Check sheet for the drawn part. Datum: minimum x, y, z corner. Units: mm. A direction names the side the tool comes from. Round coordinates to 2 decimals unless told otherwise and drop trailing zeros. Write each loop counter-clockwise with the first axis right and the second up, starting at its lowest first coordinate (ties: lowest second). Pieces come first, ordered by that corner, then holes. Notation, with made-up numbers: M 10.25,65 L 63.25,65 A14 cw 63.25,74 Z; hole C 52.5,32.25 d9. An arc over 180 degrees is marked long. Answer in a Markdown table with one row per item. Add a question column.
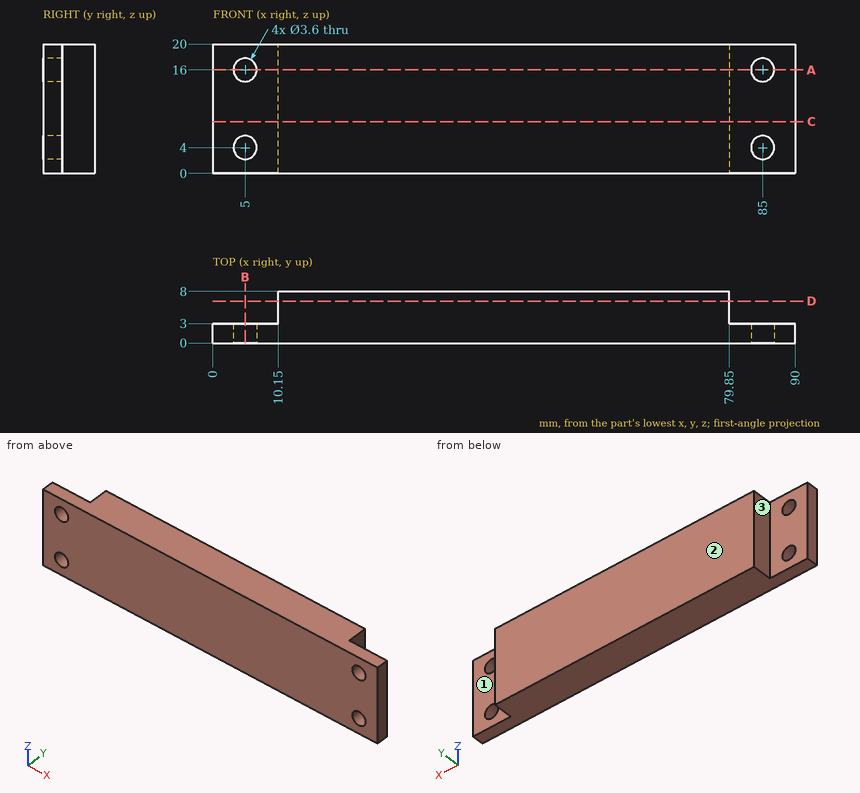
Item 1: Section check D-D, the plane y = 6.5. Record the boundary of the cut face in (x, z), and give its area (3 significant figures).
Item 2: Gauge pin test, flat ends, axial feed: pin 1 Ø2 at (x, z) = (85, 4) entering from +Y; pin 2 Ø3 at (x, z) = (85.5, 13.5) entering from +Y. Record the tip position at first contact, or that the pin passes through.
Item 3: Section check A-A, the plane z = 16. Record the boundary of the cut face in (x, y).
Item 4: Access from +Z, -Z, +X, -X, +Y, -Y to the whole of each face (thin tool, end or side, straight path). Record for the marked faces 1, 2 and 3.
Item 5: Scan lines: probe 1 along Z at (x, y) = (85, 2.35); probe 2 along X at (y, z) = (2.1, 4); probe 3 along X at (y, z) = (7.5, 2.5). Record each from-to range of solid material in increasing order. Write a range as from..to.
Item 6: Section check B-B, the plane x = 5. Record the boundary of the cut face in (y, z).
Item 7: Section check C-C, the plane z = 8. Record the boundary of the cut face in (x, y), and give its area (4 significant figures).
Result sheet:
| question | item | result |
|---|---|---|
| 1 | outline | M 10.15,0 L 79.85,0 L 79.85,20 L 10.15,20 Z |
| 1 | area | 1,390 mm^2 |
| 2 | pin 1 | passes through |
| 2 | pin 2 | stops at y = 3 |
| 3 | outline | M 0,0 L 3.2,0 L 3.2,3 L 0,3 Z; M 6.8,0 L 83.2,0 L 83.2,3 L 79.85,3 L 79.85,8 L 10.15,8 L 10.15,3 L 6.8,3 Z; M 86.8,0 L 90,0 L 90,3 L 86.8,3 Z |
| 4 | face 1 | +Z, -Z, +X, +Y |
| 4 | face 2 | +Z, -Z, +X, -X, +Y |
| 4 | face 3 | +Z, -Z, -X, +Y |
| 5 | probe 1 | z = 0..2.2, 5.8..14.2, 17.8..20 |
| 5 | probe 2 | x = 0..3.2, 6.8..83.2, 86.8..90 |
| 5 | probe 3 | x = 10.15..79.85 |
| 6 | outline | M 0,0 L 3,0 L 3,2.2 L 0,2.2 Z; M 0,5.8 L 3,5.8 L 3,14.2 L 0,14.2 Z; M 0,17.8 L 3,17.8 L 3,20 L 0,20 Z |
| 7 | outline | M 0,0 L 90,0 L 90,3 L 79.85,3 L 79.85,8 L 10.15,8 L 10.15,3 L 0,3 Z |
| 7 | area | 618.5 mm^2 |
